```python
from build123d import *

# Parameters (mm, degrees)
F0_W     = 120
F0_H     = 120
F1_DEPTH = 10
F2_R     = 4.25
F2_R_2   = 2
F3_DEPTH = 10.001
F4_R     = 2
F5_DEPTH = 10.001


with BuildPart() as f1:
    # F0 (on Front) → F1 (new body)
    with BuildSketch(Plane.XZ):
        with Locations((60, 60)):
            Rectangle(F0_W, F0_H)
    extrude(amount=F1_DEPTH)

    # F2 (on face) → F3 (cut, through all)
    with BuildSketch(Plane.XZ.offset(10)):
        with Locations((40, 100)):
            Circle(F2_R)
        with Locations((104, 100)):
            Circle(F2_R)
        with Locations((85, 110)):
            Circle(F2_R_2)
    extrude(amount=-F3_DEPTH, mode=Mode.SUBTRACT)

    # F4 (on face) → F5 (cut, through all)
    with BuildSketch(Plane.XZ.offset(10)):
        with Locations((10, 42.5)):
            Circle(F4_R)
        with Locations((10, 85)):
            Circle(F4_R)
        with Locations((70, 85)):
            Circle(F4_R)
        with Locations((70, 42.5)):
            Circle(F4_R)
    extrude(amount=-F5_DEPTH, mode=Mode.SUBTRACT)


solid = f1.part
```
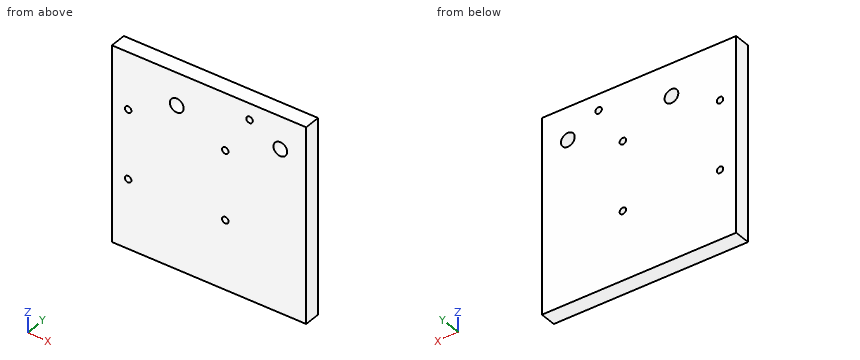
Check sheet for the modelled part. Datum: model origin and axes. Units: mm. Round coordinates to 2 decimals unless told otherwise and drop trailing zeros. Order: outer loops, then holes, each group sorted by start corner. A loop starts at its lowest first (then second) coordinate and runs counter-clockwise, first axis right, second up. Notation, with made-up numbers: (25.25, -15.5) - (48.25, -15.5) arc R16 cw to (48.25, 14.5) - close; hole circle Ø6 at (-30, 8.25). An arc over 180 degrees is marked (long way). Answer as CSV lines item,"result". Start each with the question number.
1) Section check A-A (x = 40). Record the cut outline in (y, z), then the cut area to 4 significant figures.
2) Scan lines: probe 1 along Z at (x, y) = (10, -4.5); probe 2 along Z at (x, y) = (104, -6.5); probe 3 along Z at (x, y) = (107, -1.75). Record each from-to range of solid material in increasing order.
3) Section check B-B (z = 85). Record the cut outline in (x, y), then the cut area to 3 significant figures.
4) Depth check by flat-ended pin: pin 1 (7 mm diameter, centred on x = 40, z = 100, fed in from -Y). Enter the tip coordinate at first touch or a pass-through.
5) Section check C-C (x = 10). Record the cut outline in (y, z).
6) Section check D-D (x = 85). Record the cut outline in (y, z).
Determined:
1,outline,"(-10, 0) - (0, 0) - (0, 95.75) - (-10, 95.75) - close; (-10, 104.25) - (0, 104.25) - (0, 120) - (-10, 120) - close"
1,area,"1,115 mm^2"
2,probe 1,"0 to 40.5, 44.5 to 83, 87 to 120"
2,probe 2,"0 to 95.75, 104.25 to 120"
2,probe 3,"0 to 96.99, 103.01 to 120"
3,outline,"(0, -10) - (8, -10) - (8, 0) - (0, 0) - close; (12, -10) - (68, -10) - (68, 0) - (12, 0) - close; (72, -10) - (120, -10) - (120, 0) - (72, 0) - close"
3,area,"1,120 mm^2"
4,pin 1,"through"
5,outline,"(-10, 0) - (0, 0) - (0, 40.5) - (-10, 40.5) - close; (-10, 44.5) - (0, 44.5) - (0, 83) - (-10, 83) - close; (-10, 87) - (0, 87) - (0, 120) - (-10, 120) - close"
6,outline,"(-10, 0) - (0, 0) - (0, 108) - (-10, 108) - close; (-10, 112) - (0, 112) - (0, 120) - (-10, 120) - close"
